from build123d import *

# Parameters (mm, degrees)
PAD_DEPTH    = 3.81
SKETCH001_R  = 2
PAD001_DEPTH = 5


with BuildPart() as part:
    # Sketch → Pad (new body)
    with BuildSketch(Plane.YZ):
        with BuildLine():
            Line((50.8, 7.112), (50.8, 0))
            Line((50.8, 0), (0, 0))
            Line((0, 0), (0, 7.112))
            ThreePointArc((15.621017, 14.224002), (6.878912, 12.714188), (0, 7.112))
            Line((15.621017, 14.224002), (22.479017, 14.224002))
            ThreePointArc((50.8, 7.112), (37.249044, 13.095258), (22.479017, 14.224002))
        make_face()
    extrude(amount=PAD_DEPTH)

    # Sketch001 (on Face8 of Pad) → Pad001 (join)
    with BuildSketch(Plane.YZ.offset(3.81)):
        with Locations((46.3, 2.112)):
            Circle(SKETCH001_R)
    extrude(amount=PAD001_DEPTH)


solid = part.part
Work out the finished part from the listing and answer in its coordinate system (mm). Round coordinates to 2 decimals unless told otherwise and drop trailing zeros. Loops run counter-clockwise (first coordinate to the right, second up) from the corner with the lowest first, then second, coordinate; pieces in that order, holes last. Notation, with made-up numbers: M 9.5,13 L 36.5,13 A3 ccw 36.5,17 Z; hole C 6,84 d10. An arc over 180 degrees is marked long. One line per question, with ' | ' between items. Start each with the question number.
(1) Flat-ended cylindrical pins translate along their axes: pin 1 Ø3 at (y, z) = (42.5, 8.5) entering from +X; pin 2 Ø3 at (x, y) = (2.5, 21) entering from +Z. Find the tip coordinate at first contact, or state that the pin passes through.
(2) A cutting plane is placed at B-B on y = 46.3. Write down the section's boundary in (x, z).
(3) A cutting plane is placed at C-C on z = 4.75. Write down the section's boundary in (x, y), plus the area to 3 significant figures.
(4) A cutting plane is placed at D-D on z = 10.75. Write down the section's boundary in (x, y).
(5) Find the intervals of material crossed by line 1 (Z direction, x = 3.5, y = 14.5); line 2 (X direction, y = 12, z = 9.5); line 3 (Y direction, x = 7, z = 1.25), in increasing order.
(6) For a pull along Y with two mould halves and no side action, classify faces 1 (the face through (6.28, 48.21, 2.71)), 2 (the face through (2, 19, 14.224)), 3 (the face through (8.81, 46, 2)) as released by +Y, released by -Y, zero draft, split by the parting line, or undercut.
(7) A cutting plane is placed at A-A on x = 2.75. Write down the section's boundary in (y, z).
Geometry check:
1) pin 1: stops at x = 3.81 | pin 2: stops at z = 14.23
2) outline: M 0,0 L 3.81,0 L 3.81,0.11 L 8.81,0.11 L 8.81,4.11 L 3.81,4.11 L 3.81,9.73 L 0,9.73 Z
3) outline: M 0,0 L 3.81,0 L 3.81,50.8 L 0,50.8 Z | area: 194 mm²
4) outline: M 0,3.58 L 3.81,3.58 L 3.81,44.12 L 0,44.12 Z
5) line 1: z = 0 to 14.28 | line 2: x = 0 to 3.81 | line 3: y = 44.5 to 48.1
6) face 1: split by the parting line | face 2: undercut | face 3: zero draft
7) outline: M 0,0 L 50.8,0 L 50.8,7.11 A43.84 ccw 22.48,14.22 L 15.62,14.22 A17.5 ccw 0,7.11 Z
